Autodesk Inventor part; units mm, degrees
ref_plane "YZ Plane" through (0, 0, 0) normal (1, 0, 0) x (0, 1, 0)
ref_plane "XZ Plane" through (0, 0, 0) normal (0, 1, 0) x (-1, 0, 0)
ref_plane "XY Plane" through (0, 0, 0) normal (0, 0, 1) x (1, 0, 0)
sketch "Sketch1" plane through (0, 0, 0) normal (0, 0, 1) x (1, 0, 0)
  circle A0 centre (0, 0) radius 194.5
  circle A1 centre (0, 0) radius 234.5
  dimension "d0" = 40
  dimension "d1" = 389
extrude "Extrusion1" add sketch "Sketch1" along normal blind 38
sketch "Sketch2" plane through (0, 0, 38) normal (0, 0, 1) x (1, 0, 0)
  circle A0 centre (0, 0) radius 234.5 construction
  circle A1 centre (0, 0) radius 194.5 construction
  line L0 (0, 234.5) -> (0, 194.5) construction
  circle A2 centre (0, 214.5) radius 6.25
  dimension "d4" = 12.5
extrude "Extrusion2" cut sketch "Sketch2" against normal through all
sketch "Sketch3" plane through (0, 0, 38) normal (0, 0, 1) x (1, 0, 0)
  circle A0 centre (0, 214.5) radius 6.25
  circle A1 centre (0, 214.5) radius 13.75
  point P0 (0, 0)
  dimension "d10" = 27.5
extrude "Extrusion3" cut sketch "Sketch3" against normal blind 11
pattern_circular "Circular Pattern1" count 8 over 360 about axis through (0, 0, 0) along (0, 0, 1) of "Extrusion2", "Extrusion3"
sketch "Sketch4" plane through (0, 0, 0) normal (0, 0, -1) x (-1, 0, 0)
  circle A0 centre (0, 0) radius 234.5
  circle A1 centre (0, 0) radius 239.5
  dimension "d13" = 5
extrude "Extrusion4" add sketch "Sketch4" against normal blind 9
sketch "Sketch5" plane through (0, 0, 0) normal (1, 0, 0) x (0, 1, 0)
  line L0 (234.5, 9) -> (234.5, 38)
  line L1 (239.5, 9) -> (-239.5, 9)
  line L2 (239.5, 0) -> (239.5, 9)
  line L3 (-239.5, 0) -> (239.5, 0)
  line L4 (-234.5, 9) -> (-234.5, 38)
  line L5 (-239.5, 0) -> (-239.5, 9)
  line L6 (-234.5, 19) -> (234.5, 19)
  line L7 (234.5, 38) -> (-234.5, 38)
  line L8 (234.5, 38) -> (-234.5, 38)
  point P0 (0, 0)
  dimension "d16" = 38
  dimension "d17" = 19
extrude "Extrusion5" cut sketch "Sketch5" along normal through all both and the other way through all contours L6 L4 L7 L0
equation "\"d1\" = Вал_ось_диаметр_КОРМА"
equation "\"BendRadius\" = Thickness"
equation "\"BendReliefWidth\" = Thickness"
equation "\"BendReliefDepth\" = 0.5 * Thickness"
equation "\"CornerReliefSize\" = 4 * Thickness"
equation "\"MinimumRemnant\" = 2 * Thickness"
equation "\"TransitionRadius\" = BendRadius"
equation "\"JacobiRadiusSize\" = BendRadius"
equation "\"GapSize\" = Thickness"
properties part number "ДМФ 01 32.2 Барабан Опорное кольцо КОРМА"
Verification items for the finished model (mm, model axes). A direction names the side the tool comes from. Coordinates: 2 decimals unless noted, no trailing zeros. Write each loop counter-clockwise with the first axis right and the second up, starting at its lowest first coordinate (ties: lowest second). Pieces come first, ordered by that corner, then holes. Notation, with made-up numbers: (56.5, 51) -> (68.5, 51) arc R4 cw to (68.5, 56) -> close; hole circle Ø1 at (67.25, 80). An arc over 180 degrees is marked (long way). One line per item, written item: value. Start each with the question number.
Q1. Mould release check, pull along X, two halves, no side actions. Record for faces 3 (the cylindrical face through (148.32, -146.4, 9.63)), 4 (the flat face through (-176, -159, 9)), 5 (the cylindrical face through (31.18, 237.46, 4.44)): pulls with the +X half, pulls with the -X half, needs draft (parallel to the pull), parting line crosses it, or undercut.
Q2. Cross-section at C-C on y = 124.5. Enter the section's corners in (x, z).
Q3. Access from +Z, -Z, +X, -X, +Y, -Y to the whole of each face (thin tool, end or side, straight path). Record for faces 1 (the cylindrical face through (223.67, -70.44, 13.93)), 2 (the cylindrical face through (-42.164, 189.875, 9.367)).
Q4. Cross-section at D-D on x = -214.5. Enter the section's corners in (y, z).
Q5. Thickness scan on L1, parallel to Y at x = 0, z = 5; L2, parallel to X at y = -5.5, z = 17.75; L3, parallel to X at y = 132.5, z = 14.25. Record the ranges inside material, lowest first. Write a range as from..to.
Q6. Cross-section at A-A on x = 0. Enter the section's corners in (y, z), and give its area (4 significant figures).
Q7. Go/stop test with flat-tipped pins: P1, Ø5, axis at x = -35.5, z = 3, coming from the +Y side; P2, Ø1, axis at y = -164, z = 6, coming from the +X side; P3, Ø1.5, axis at x = -156, z = 16.5, coming from the +Y side. Record where each tip stops, or that it passes through.
Checked values:
1. face 3: undercut
1. face 4: needs draft
1. face 5: parting line crosses it
2. outline: (-204.6, 0) -> (-149.43, 0) -> (-149.43, 19) -> (-198.72, 19) -> (-198.72, 9) -> (-204.6, 9) -> close; (149.43, 0) -> (204.6, 0) -> (204.6, 9) -> (198.72, 9) -> (198.72, 19) -> (149.43, 19) -> close
3. face 1: +Z
3. face 2: +Z, -Z
4. outline: (-106.54, 0) -> (-6.25, 0) -> (-6.25, 19) -> (-94.76, 19) -> (-94.76, 9) -> (-106.54, 9) -> close; (6.25, 0) -> (106.54, 0) -> (106.54, 9) -> (94.76, 9) -> (94.76, 19) -> (6.25, 19) -> close
5. L1: y = -239.5..-220.75, -208.25..-194.5, 194.5..208.25, 220.75..239.5
5. L2: x = -234.44..-217.47, -211.53..-194.42, 194.42..211.53, 217.47..234.44
5. L3: x = -193.48..-142.39, 142.39..193.48
6. outline: (-239.5, 0) -> (-220.75, 0) -> (-220.75, 19) -> (-234.5, 19) -> (-234.5, 9) -> (-239.5, 9) -> close; (-208.25, 0) -> (-194.5, 0) -> (-194.5, 19) -> (-208.25, 19) -> close; (194.5, 0) -> (208.25, 0) -> (208.25, 19) -> (194.5, 19) -> close; (220.75, 0) -> (239.5, 0) -> (239.5, 9) -> (234.5, 9) -> (234.5, 19) -> (220.75, 19) -> close
6. area: 1,135 mm²
7. P1: stops at y = 237.22
7. P2: stops at x = 175.01
7. P3: stops at y = 175.75
